from build123d import *

# Parameters (mm, degrees)
CYLINDER_R     = 2
CYLINDER_DEPTH = 10
SKETCH_R       = 2.5
EXTRUDE_DEPTH  = 5


with BuildPart() as pin:
    # Cylinder → Cylinder (new body)
    with BuildSketch(Plane(origin=(10, 0, 0), x_dir=(1, 0, 0), z_dir=(0, 0, 1))):
        Circle(CYLINDER_R)
    extrude(amount=CYLINDER_DEPTH)


with BuildPart() as fusion:
    # Sketch → Extrude (new body)
    with BuildSketch(Plane.XY):
        with BuildLine():
            ThreePointArc((0, 5), (-5, 0), (0, -5))
            Line((0, -5), (10, -5))
            ThreePointArc((10, -5), (15, 0), (10, 5))
            Line((0, 5), (10, 5))
        make_face()
        Circle(SKETCH_R, mode=Mode.SUBTRACT)
    extrude(amount=EXTRUDE_DEPTH)

    # Fusion: union Pin
    add(pin.part)


solid = fusion.part
Verification items for the finished model (mm, model axes). A direction names the side the tool comes from. Coordinates: 2 decimals unless noted, no trailing zeros. Order: outer loops, then holes, each group sorted by start corner. A loop starts at its lowest first (then second) coordinate and runs counter-clockwise, first axis right, second up.
Item 1: Material ranges on L1, parallel to Y at x = 0, z = 1.3; L2, parallel to Z at x = 1.25, y = -2.75; L3, parallel to Y at x = 10, z = 9.5, recorded low to high.
Filled in:
L1: y = -5 to -2.5, 2.5 to 5
L2: z = 0 to 5
L3: y = -2 to 2
Item 2: Depth check by flat-ended pin: pin 1 (3 mm diameter, centred on x = 0, y = 0, fed in from -Z); pin 2 (4 mm diameter, centred on y = -3.5, z = 7.5, fed in from -X); pin 3 (4 mm diameter, centred on y = 0.5, z = 8.5, fed in from +X); pin 4 (4 mm diameter, centred on y = -2.5, z = 6.5, fed in from -X). Enter the tip coordinate at first touch or a pass-through.
Filled in:
pin 1: passes through
pin 2: stops at x = 8.68
pin 3: stops at x = 12
pin 4: stops at x = -4.86
Item 3: Section check C-C, the plane z = 4. Enter the section's corners in (x, y).
Filled in:
outline: (0, -5) - (10, -5) arc R5 ccw to (10, 5) - (0, 5) arc R5 ccw to start; hole circle Ø5 at (0, 0)
Item 4: Section check A-A, the plane y = 0. Enter the section's corners in (x, z).
Filled in:
outline: (-5, 0) - (-2.5, 0) - (-2.5, 5) - (-5, 5) - close; (2.5, 0) - (15, 0) - (15, 5) - (12, 5) - (12, 10) - (8, 10) - (8, 5) - (2.5, 5) - close
Item 5: Access from +Z, -Z, +X, -X, +Y, -Y to the whole of each face (thin tool, end or side, straight path). Record for faces 1 (the face through (5, 5, 2)), 2 (the face through (8.4, -1.2, 7.5)).
Filled in:
face 1: +Z, -Z, +X, -X, +Y
face 2: +Z
Item 6: Section check B-B, the plane x = 1.5. Enter the section's corners in (y, z).
Filled in:
outline: (-5, 0) - (-2, 0) - (-2, 5) - (-5, 5) - close; (2, 0) - (5, 0) - (5, 5) - (2, 5) - close
Item 7: Section check D-D, the plane x = 5.5. Enter the section's corners in (y, z).
Filled in:
outline: (-5, 0) - (5, 0) - (5, 5) - (-5, 5) - close
